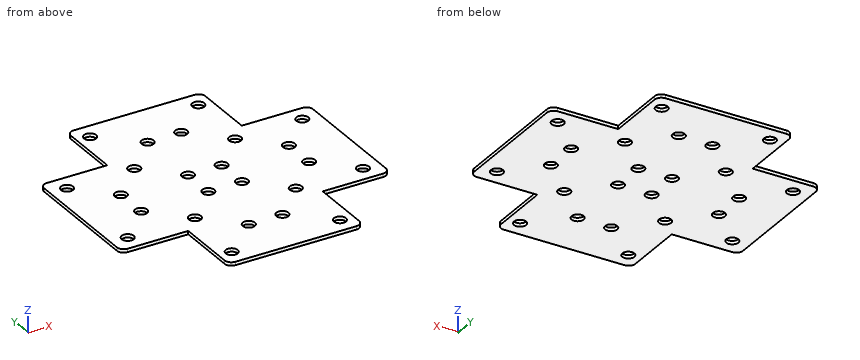
from build123d import *

# Parameters (mm, degrees)
F1_DEPTH = 5
F2_R     = 9
F3_DEPTH = 25
F4_R     = 10


with BuildPart() as f1:
    # F0 (on Top) → F1 (new body)
    with BuildSketch(Plane.XY):
        Polygon((-100, -200), (0, -200), (100, -200), (100, -100), (200, -100), (200, 0), (200, 100), (100, 100), (100, 200), (0, 200), (-100, 200), (-100, 100), (-200, 100), (-200, 0), (-200, -100), (-100, -100), align=None)
    extrude(amount=F1_DEPTH)

    # F2 (on face) → F3 (cut)
    with BuildSketch(Plane.XY.offset(5)):
        with Locations((25, 25)):
            Circle(F2_R)
        with Locations((75, 75)):
            Circle(F2_R)
        with Locations((125, 25)):
            Circle(F2_R)
        with Locations((175, 75)):
            Circle(F2_R)
        with Locations((25, 125)):
            Circle(F2_R)
        with Locations((80.500526, 175)):
            Circle(F2_R)
        with Locations((80.500526, -175)):
            Circle(F2_R)
        with Locations((25, -125)):
            Circle(F2_R)
        with Locations((175, -75)):
            Circle(F2_R)
        with Locations((75, -75)):
            Circle(F2_R)
        with Locations((125, -25)):
            Circle(F2_R)
        with Locations((25, -25)):
            Circle(F2_R)
        with Locations((-25, -125)):
            Circle(F2_R)
        with Locations((-175, 75)):
            Circle(F2_R)
        with Locations((-175, -75)):
            Circle(F2_R)
        with Locations((-80.500526, 175)):
            Circle(F2_R)
        with Locations((-25, 25)):
            Circle(F2_R)
        with Locations((-125, 25)):
            Circle(F2_R)
        with Locations((-125, -25)):
            Circle(F2_R)
        with Locations((-80.500526, -175)):
            Circle(F2_R)
        with Locations((-25, -25)):
            Circle(F2_R)
        with Locations((-25, 125)):
            Circle(F2_R)
        with Locations((-75, 75)):
            Circle(F2_R)
        with Locations((-75, -75)):
            Circle(F2_R)
    extrude(amount=-F3_DEPTH, mode=Mode.SUBTRACT)

    # F4
    f4_edges = [f1.edges().sort_by_distance(p)[0] for p in [
        (100, -200, 2.5),
        (-100, -200, 2.5),
        (-200, -100, 2.5),
        (-200, 100, 2.5),
        (-100, 200, 2.5),
        (100, 200, 2.5),
        (200, 100, 2.5),
        (200, -100, 2.5),
    ]]
    fillet(f4_edges, radius=F4_R)


solid = f1.part
Verification items for the finished model (mm, model axes). Coordinates: 2 decimals unless noted, no trailing zeros. Order: outer loops, then holes, each group sorted by start corner. A loop starts at its lowest first (then second) coordinate and runs counter-clockwise, first axis right, second up.
Item 1: Section check C-C, the plane y = -175. Enter the section's corners in (x, z), then the cut area to 3 significant figures.
Filled in:
outline: (-100, 0) - (-89.5, 0) - (-89.5, 5) - (-100, 5) - close; (-71.5, 0) - (71.5, 0) - (71.5, 5) - (-71.5, 5) - close; (89.5, 0) - (100, 0) - (100, 5) - (89.5, 5) - close
area: 820 mm2
Item 2: Section check A-A, the plane y = 75. Enter the section's corners in (x, z).
Filled in:
outline: (-200, 0) - (-184, 0) - (-184, 5) - (-200, 5) - close; (-166, 0) - (-84, 0) - (-84, 5) - (-166, 5) - close; (-66, 0) - (66, 0) - (66, 5) - (-66, 5) - close; (84, 0) - (166, 0) - (166, 5) - (84, 5) - close; (184, 0) - (200, 0) - (200, 5) - (184, 5) - close
Item 3: Depth check by flat-ended pin: pin 1 (2.5 mm diameter, centred on y = 129.5, z = 1.5, fed in from -X); pin 2 (1.5 mm diameter, centred on y = -152.5, z = 3.5, fed in from +X); pin 3 (1.5 mm diameter, centred on x = 132.5, y = 49, fed in from -Z); pin 4 (11 mm diameter, centred on x = 125, y = 25, fed in from +Z). Enter the tip coordinate at first touch or a pass-through.
Filled in:
pin 1: stops at x = -100
pin 2: stops at x = 100
pin 3: stops at z = 0
pin 4: passes through
Item 4: Section check B-B, the plane x = 125. Enter the section's corners in (y, z), then the cut area to 3 significant figures.
Filled in:
outline: (-100, 0) - (-34, 0) - (-34, 5) - (-100, 5) - close; (-16, 0) - (16, 0) - (16, 5) - (-16, 5) - close; (34, 0) - (100, 0) - (100, 5) - (34, 5) - close
area: 820 mm2
Item 5: Material ranges on L1, parallel to Y at x = -24.5, z = 4.1; L2, parallel to Y at x = 125, z = 1.9; L3, parallel to Y at x = 175, z = 1.2, recorded low to high.
Filled in:
L1: y = -200 to -133.99, -116.01 to -33.99, -16.01 to 16.01, 33.99 to 116.01, 133.99 to 200
L2: y = -100 to -34, -16 to 16, 34 to 100
L3: y = -100 to -84, -66 to 66, 84 to 100
Item 6: Section check D-D, the plane x = 25. Enter the section's corners in (y, z).
Filled in:
outline: (-200, 0) - (-134, 0) - (-134, 5) - (-200, 5) - close; (-116, 0) - (-34, 0) - (-34, 5) - (-116, 5) - close; (-16, 0) - (16, 0) - (16, 5) - (-16, 5) - close; (34, 0) - (116, 0) - (116, 5) - (34, 5) - close; (134, 0) - (200, 0) - (200, 5) - (134, 5) - close
